Geometry check sheet. Reference: the model listing, model coordinates, mm. Face numbers are marked on the shaded views. Coordinates: 2 decimals unless noted, no trailing zeros. Loops run counter-clockwise (first coordinate to the right, second up) from the corner with the lowest first, then second, coordinate; pieces in that order, holes last. Notation, with made-up numbers: (-7.75, 37) -> (44.25, 37) arc R27 cw to (44.25, 61) -> close; hole circle Ø8 at (67, 43). An arc over 180 degrees is marked (long way). Answer as a JSON object with one key per item and string values.
from build123d import *

# Parameters (mm, degrees)
SKETCH1_W           = 60.325
SKETCH1_H           = 12.7
SKETCH1_R           = 2.159
BOSS_EXTRUDE1_DEPTH = 12.7
SKETCH5_R           = 3.556
CUT_EXTRUDE1_DEPTH  = 3.81
FILLET1_R           = 0.762


with BuildPart() as part:
    # Sketch1 → Boss-Extrude1 (new body)
    with BuildSketch(Plane(origin=(0, 0, 0), x_dir=(1, 0, 0), z_dir=(0, 1, 0))):
        with Locations((30.1625, 6.35)):
            Rectangle(SKETCH1_W, SKETCH1_H)
        with Locations((17.4625, 6.35)):
            Circle(SKETCH1_R, mode=Mode.SUBTRACT)
        with Locations((42.8625, 6.35)):
            Circle(SKETCH1_R, mode=Mode.SUBTRACT)
    extrude(amount=BOSS_EXTRUDE1_DEPTH)

    # Sketch5 → Cut-Extrude1 (cut)
    with BuildSketch(Plane.XZ):
        with Locations((42.8625, -6.35)):
            Circle(SKETCH5_R)
        with Locations((17.4625, -6.35)):
            Circle(SKETCH5_R)
    extrude(amount=-CUT_EXTRUDE1_DEPTH, mode=Mode.SUBTRACT)

    # Fillet1
    fillet1_edges = [part.edges().sort_by_distance(p)[0] for p in [
        (60.325, 12.7, -6.35),
        (30.1625, 12.7, -12.7),
        (39.3065, 0, -6.35),
        (13.9065, 0, -6.35),
        (0, 12.7, -6.35),
        (30.1625, 0, -12.7),
        (60.325, 0, -6.35),
        (30.1625, 0, 0),
        (0, 0, -6.35),
        (30.1625, 12.7, 0),
        (0, 6.35, -12.7),
        (60.325, 6.35, -12.7),
        (60.325, 6.35, 0),
        (0, 6.35, 0),
    ]]
    fillet(fillet1_edges, radius=FILLET1_R)


solid = part.part
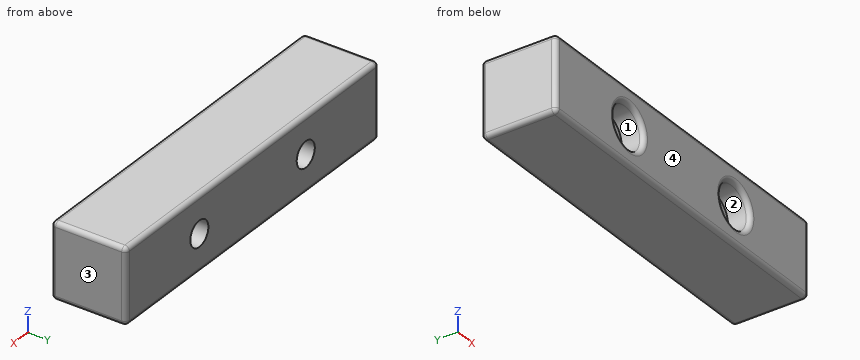
1. Section check B-B, the plane y = 6.75. State how many separate pieces and enclosed holes the cut face has, then the cut area to 3 significant figures.
Evaluation:
{"separate pieces": "1", "enclosed holes": "2", "area": "736 mm^2"}
2. Mould release check, pull along X, two halves, no side actions. Record for the marked faces 1, 2, 3 and 4: released by +X, released by -X, zero draft, split by the parting line, or undercut.
Evaluation:
{"face 1": "undercut", "face 2": "undercut", "face 3": "released by +X", "face 4": "zero draft"}
3. Depth check by flat-ended pin: P1, Ø2, axis at x = 40, z = -10, coming from the -Y side; P2, Ø6.5, axis at x = 42.86, z = -6.35, coming from the -Y side. Enter the tip coordinate at first touch or a pass-through.
Evaluation:
{"P1": "stops at y = 0", "P2": "stops at y = 3.81"}
4. Thickness scan on probe 1 along X at (y, z) = (11, -6.35) (1 decimal); probe 2 along X at (y, z) = (7.75, -4.5) (1 decimal); probe 3 along Y at (x, z) = (14, -6.25). Record the ranges inside material, lowest first. Write a range as from..to.
Evaluation:
{"probe 1": "x = 0..15.3, 19.6..40.7, 45..60.3", "probe 2": "x = 0..16.3, 18.6..41.7, 44..60.3", "probe 3": "y = 3.81..12.7"}
5. Section check A-A, the plane z = -6.35. Record the boundary of the cut face in (x, y) (1 decimal), then the cut area to 3 significant figures.
Evaluation:
{"outline": "(0, 0.8) arc R0.8 ccw to (0.8, 0) -> (13.1, 0) arc R0.8 ccw to (13.9, 0.8) -> (13.9, 3.8) -> (15.3, 3.8) -> (15.3, 12.7) -> (0.8, 12.7) arc R0.8 ccw to (0, 11.9) -> close; (19.6, 3.8) -> (21, 3.8) -> (21, 0.8) arc R0.8 ccw to (21.8, 0) -> (38.5, 0) arc R0.8 ccw to (39.3, 0.8) -> (39.3, 3.8) -> (40.7, 3.8) -> (40.7, 12.7) -> (19.6, 12.7) -> close; (45, 3.8) -> (46.4, 3.8) -> (46.4, 0.8) arc R0.8 ccw to (47.2, 0) -> (59.6, 0) arc R0.8 ccw to (60.3, 0.8) -> (60.3, 11.9) arc R0.8 ccw to (59.6, 12.7) -> (45, 12.7) -> close", "area": "634 mm^2"}
